from build123d import *

# Parameters (mm, degrees)
SKETCH1_W           = 10.541
SKETCH1_H           = 30.734
BOSS_EXTRUDE1_DEPTH = 20.4724
SKETCH2_W           = 14.0208
SKETCH2_H           = 31.9532
BOSS_EXTRUDE2_DEPTH = 2.0066
SKETCH3_W           = 8.382
SKETCH3_H           = 23.7998
BOSS_EXTRUDE3_DEPTH = 6.35
SKETCH4_W           = 6.35
SKETCH4_H           = 0.8382
BOSS_EXTRUDE4_DEPTH = 9.144


with BuildPart() as part:
    # Sketch1 → Boss-Extrude1 (new body)
    with BuildSketch(Plane(origin=(0, 0, 0), x_dir=(1, 0, 0), z_dir=(0, 1, 0))):
        with Locations((5.2705, 15.367)):
            Rectangle(SKETCH1_W, SKETCH1_H)
    extrude(amount=BOSS_EXTRUDE1_DEPTH)

    # Sketch2 → Boss-Extrude2 (add)
    with BuildSketch(Plane(origin=(0, 20.4724, 0), x_dir=(1, 0, 0), z_dir=(0, 1, 0))):
        with Locations((5.2705, 15.367)):
            Rectangle(SKETCH2_W, SKETCH2_H)
    extrude(amount=BOSS_EXTRUDE2_DEPTH)

    # Sketch3 → Boss-Extrude3 (add)
    with BuildSketch(Plane(origin=(0, 22.479, 0), x_dir=(1, 0, 0), z_dir=(0, 1, 0))):
        with Locations((5.2705, 15.367)):
            Rectangle(SKETCH3_W, SKETCH3_H)
    extrude(amount=BOSS_EXTRUDE3_DEPTH)

    # Sketch4 → Boss-Extrude4 (add)
    with BuildSketch(Plane.XZ):
        with Locations((5.2705, -23.913230798)):
            Rectangle(SKETCH4_W, SKETCH4_H)
        with Locations((5.2705, -15.367)):
            Rectangle(SKETCH4_W, SKETCH4_H)
        with Locations((5.2705, -6.820769202)):
            Rectangle(SKETCH4_W, SKETCH4_H)
    extrude(amount=BOSS_EXTRUDE4_DEPTH)


solid = part.part
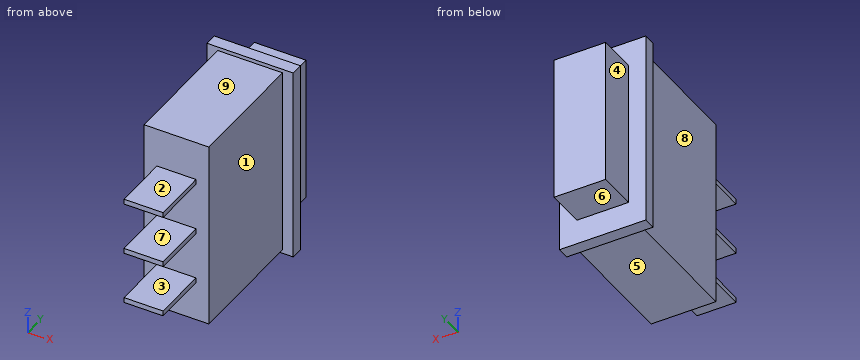
The model under review builds one solid part; all positions refer to its coordinate system, in mm. Face numbers are marked on the shaded views. A direction names the side the tool comes from. Round coordinates to 2 decimals unless told otherwise and drop trailing zeros. Write each loop counter-clockwise with the first axis right and the second up, starting at its lowest first coordinate (ties: lowest second). Pieces come first, ordered by that corner, then holes. Notation, with made-up numbers: M -31.5,38 L 21.5,38 A9 ccw 21.5,42 Z; hole C 31.5,59 d9. An arc over 180 degrees is marked long. Use a Markdown table: item, result. Add a question column.
Q1. Insertion check: pin 1 (5 mm diameter, centred on x = 9, y = 3, fed in from +Z); pin 2 (5 mm diameter, centred on x = 6.5, y = -5, fed in from +Z); pin 3 (8 mm diameter, centred on x = 3, y = 1.5, fed in from -Z). Each pin has a flat end and moves straight along its axis. Give the tip position at first contact, or say it passes through.
Q2. We need section D-D, the plane y = 26. State the section outline as (x, z) points, plus the area to 3 significant figures.
Q3. To check wall thickness, follow line 1 (Y direction, x = 6, z = -13); line 2 (Z direction, x = 2, y = 9); line 3 (X direction, y = 17, z = -6). State the ranges of each line that lie inside material, in increasing order.
Q4. We need section C-C, the plane y = 19. State the section outline as (x, z) points, plus the area to 3 significant figures.
Q5. We need section B-B, the plane x = 3.5. State the section outline as (y, z) points, plus the area to 3 significant figures.
Q6. Machinability: for the marked faces 1, 2, 3, 4 and 5, which of the approach directions +Z, -Z, +X, -X, +Y, -Y give a long, thin tool a straight path to every point of the face, cutting with its end or side? Answer none if there is none.
Q7. We need section A-A, the plane z = -25.5. State the section outline as (x, y) points.
Q8. The part is to be moulded in two halves that separate along Z. For the marked faces 6, 7, 8 and 9, say which applies: pulls with the +Z half, pulls with the -Z half, needs draft (parallel to the pull), parting line crosses it, or undercut.
Findings below:
| question | item | result |
|---|---|---|
| 1 | pin 1 | stops at z = 0 |
| 1 | pin 2 | stops at z = -6.4 |
| 1 | pin 3 | stops at z = -30.73 |
| 2 | outline | M 1.08,-27.27 L 9.46,-27.27 L 9.46,-3.47 L 1.08,-3.47 Z |
| 2 | area | 199 mm² |
| 3 | line 1 | y = 0 to 28.83 |
| 3 | line 2 | z = -30.73 to 0 |
| 3 | line 3 | x = 0 to 10.54 |
| 4 | outline | M 0,-30.73 L 10.54,-30.73 L 10.54,0 L 0,0 Z |
| 4 | area | 324 mm² |
| 5 | outline | M -9.14,-24.33 L 0,-24.33 L 0,-30.73 L 20.47,-30.73 L 20.47,-31.34 L 22.48,-31.34 L 22.48,-27.27 L 28.83,-27.27 L 28.83,-3.47 L 22.48,-3.47 L 22.48,0.61 L 20.47,0.61 L 20.47,0 L 0,0 L 0,-6.4 L -9.14,-6.4 L -9.14,-7.24 L 0,-7.24 L 0,-14.95 L -9.14,-14.95 L -9.14,-15.79 L 0,-15.79 L 0,-23.49 L -9.14,-23.49 Z |
| 5 | area | 867 mm² |
| 6 | face 1 | +Z, -Z, +X, -Y |
| 6 | face 2 | +Z, +X, -X, -Y |
| 6 | face 3 | +X, -X, -Y |
| 6 | face 4 | +Z, -Z, -X, +Y |
| 6 | face 5 | -Z, +X, -X, -Y |
| 7 | outline | M -1.74,20.47 L 0,20.47 L 0,0 L 10.54,0 L 10.54,20.47 L 12.28,20.47 L 12.28,22.48 L 9.46,22.48 L 9.46,28.83 L 1.08,28.83 L 1.08,22.48 L -1.74,22.48 Z |
| 8 | face 6 | pulls with the -Z half |
| 8 | face 7 | undercut |
| 8 | face 8 | needs draft |
| 8 | face 9 | pulls with the +Z half |
